Check sheet for the drawn part. Datum: minimum x, y, z corner. Units: mm. A direction names the side the tool comes from. Round coordinates to 2 decimals unless told otherwise and drop trailing zeros. Order: outer loops, then holes, each group sorted by start corner. A loop starts at its lowest first (then second) coordinate and runs counter-clockwise, first axis right, second up. Notation, with made-up numbers: M -29,87 L 6,87 A26 cw 6,110 Z; hole C 13.5,13 d10. An arc over 180 degrees is marked long. Answer as a JSON object with one key per item and string values. Group by question number.
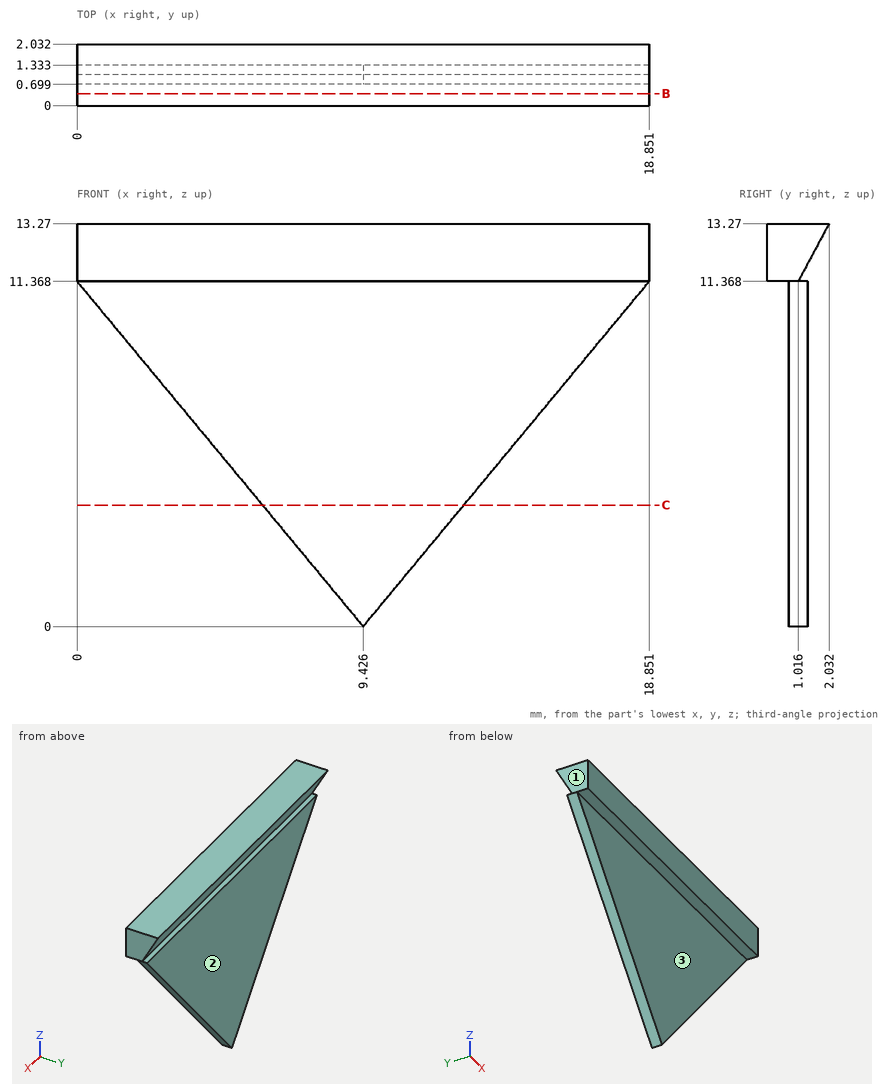
1) Set-up check for the marked faces 1, 2 and 3: record each of +Z, -Z, +X, -X, +Y, -Y from which the full face is reachable in a straight line by a thin tool's end or side.
2) Sectioned sample at B-B (y = 0.4). Record the boundary of the cut face in (x, z).
3) Sectioned sample at C-C (z = 4). Record the boundary of the cut face in (x, y).
4) Thickness scan on line 1 along Z through (x, y) = (1.75, 1.25) (1 decimal); line 2 along Y through (x, z) = (10.5, 9.5); line 3 along Z through (x, y) = (2.5, 0.1). Record the ranges inside material, lowest first. Write a range as [from, to].
5) Go/stop test with flat-tipped pins: P1, Ø2, axis at x = 11.5, z = 10, coming from the +Y side; P2, Ø3.5, axis at x = 7, z = 8.5, coming from the -Y side. Record where each tip stops, or that it passes through.
Final values:
{
 "1": {"face 1": "+Z, -Z, -X, +Y, -Y", "face 2": "-Z, +X, -X, +Y", "face 3": "-Z, +X, -X, -Y"},
 "2": {"outline": "M 0,11.37 L 18.85,11.37 L 18.85,13.27 L 0,13.27 Z"},
 "3": {"outline": "M 6.11,0.7 L 12.74,0.7 L 12.74,1.33 L 6.11,1.33 Z"},
 "4": {"line 1": "z = [9.3, 11.4], [11.8, 13.3]", "line 2": "y = [0.7, 1.33]", "line 3": "z = [11.37, 13.27]"},
 "5": {"P1": "stops at y = 1.33", "P2": "stops at y = 0.7"}
}
